```python
from build123d import *

# Parameters (mm, degrees)
SKETCH_1_W          = 35
SKETCH_1_H          = 35
SKETCH_1_R          = 1.7
EXTRUDE_1_DEPTH     = 8
SKETCH_2_W          = 5
SKETCH_2_H          = 8
EXTRUDE_2_DEPTH     = 40
SKETCH_3_R          = 1.6
CUT_EXTRUDE_1_DEPTH = 40
CUT_EXTRUDE_2_DEPTH = 24


with BuildPart() as part:
    # 草图1 → 凸台-拉伸1 (new body)
    with BuildSketch(Plane.XY):
        with Locations((6.7, -6.931428571)):
            Rectangle(SKETCH_1_W, SKETCH_1_H)
        with Locations((-4.8, 4.568571429)):
            Circle(SKETCH_1_R, mode=Mode.SUBTRACT)
        with Locations((18.2, 4.568571429)):
            Circle(SKETCH_1_R, mode=Mode.SUBTRACT)
        with Locations((-4.8, -18.431428571)):
            Circle(SKETCH_1_R, mode=Mode.SUBTRACT)
        with Locations((18.2, -18.431428571)):
            Circle(SKETCH_1_R, mode=Mode.SUBTRACT)
    extrude(amount=EXTRUDE_1_DEPTH)

    # 草图2 → 凸台-拉伸2 (add)
    with BuildSketch(Plane.XY.offset(8)):
        with Locations((-1.8, -6.931428571)):
            Rectangle(SKETCH_2_W, SKETCH_2_H)
        with Locations((15.2, -6.931428571)):
            Rectangle(SKETCH_2_W, SKETCH_2_H)
    extrude(amount=EXTRUDE_2_DEPTH)

    # 草图3 → 切除-拉伸1 (cut)
    with BuildSketch(Plane(origin=(17.7, 0, 0), x_dir=(0, 0, -1), z_dir=(1, 0, 0))):
        with Locations(Location((-38, -6.931428571, 0), (0, 0, 90))):
            Circle(SKETCH_3_R)
        with Locations(Location((-24, -6.931428571, 0), (0, 0, 90))):
            Circle(SKETCH_3_R)
    extrude(amount=-CUT_EXTRUDE_1_DEPTH, mode=Mode.SUBTRACT)

    # 草图5 → 切除-拉伸2 (cut)
    with BuildSketch(Plane.ZY.offset(4.3)):
        with BuildLine():
            Line((10.5, -6.931428571), (12, -6.931428571))
            Line((12, -6.931428571), (13.5, -6.931428571))
            ThreePointArc((13.5, -6.931428571), (12, -5.431428571), (10.5, -6.931428571))
        make_face()
        with BuildLine():
            Line((13.5, -6.931428571), (12, -6.931428571))
            Line((12, -6.931428571), (10.5, -6.931428571))
            ThreePointArc((10.5, -6.931428571), (12, -8.431428571), (13.5, -6.931428571))
        make_face()
        with BuildLine():
            ThreePointArc((45.5, -6.931428571), (44, -5.431428571), (42.5, -6.931428571))
            Line((42.5, -6.931428571), (44, -6.931428571))
            Line((44, -6.931428571), (45.5, -6.931428571))
        make_face()
        with BuildLine():
            Line((44, -6.931428571), (42.5, -6.931428571))
            ThreePointArc((42.5, -6.931428571), (44, -8.431428571), (45.5, -6.931428571))
            Line((45.5, -6.931428571), (44, -6.931428571))
        make_face()
    extrude(amount=-CUT_EXTRUDE_2_DEPTH, mode=Mode.SUBTRACT)


solid = part.part
```
Build history of the part. All positions in model axes, mm. A direction names the side the tool comes from. Round coordinates to 2 decimals unless told otherwise and drop trailing zeros. Order: outer loops, then holes, each group sorted by start corner. A loop starts at its lowest first (then second) coordinate and runs counter-clockwise, first axis right, second up. Notation, with made-up numbers: (73, 71.5) -> (88, 71.5) arc R21 cw to (88, 98.5) -> close; hole circle Ø3 at (15, -15). An arc over 180 degrees is marked (long way). Answer in a Markdown table with one row per item.
1) Wall check: L1, parallel to X at y = -4.5, z = 28.5; L2, parallel to Y at x = -4.8, z = 5; L3, parallel to Z at x = 5, y = -14.5. Give the ranges that are in metal, low to high.
Values:
| item | result |
|---|---|
| L1 | -4.3 to 0.7, 12.7 to 17.7 |
| L2 | -24.43 to -20.13, -16.73 to 2.87, 6.27 to 10.57 |
| L3 | 0 to 8 |
2) Band-saw the part on D-D on x = 13.5. Give the cut face in (y, z).
Values:
| item | result |
|---|---|
| outline | (-24.43, 0) -> (10.57, 0) -> (10.57, 8) -> (-2.93, 8) -> (-2.93, 48) -> (-10.93, 48) -> (-10.93, 8) -> (-24.43, 8) -> close; hole circle Ø3.2 at (-6.93, 24); hole circle Ø3.2 at (-6.93, 38); hole circle Ø3 at (-6.93, 12); hole circle Ø3 at (-6.93, 44) |
3) Band-saw the part on B-B on z = 35.5. Give the cut face in (x, y).
Values:
| item | result |
|---|---|
| outline | (-4.3, -10.93) -> (0.7, -10.93) -> (0.7, -2.93) -> (-4.3, -2.93) -> close; (12.7, -10.93) -> (17.7, -10.93) -> (17.7, -2.93) -> (12.7, -2.93) -> close |
4) Which spindle directions (+Z, -Z, +X, -X, +Y, -Y) get a long thin tool onto all of the face, cutting with end or side? Do faces 4 (the flat face through (0.7, -7, 28)), 5 (the flat face through (15, -2.931, 28)), 6 (the flat face through (-2, -10.931, 28)). Say none if no direction does.
Values:
| item | result |
|---|---|
| face 4 | +Z, +Y, -Y |
| face 5 | +Z, +X, -X, +Y |
| face 6 | +Z, +X, -X, -Y |
5) Band-saw the part on A-A on z = 24. Give the cut face in (x, y), and give its area (3 significant figures).
Values:
| item | result |
|---|---|
| outline | (-4.3, -10.93) -> (0.7, -10.93) -> (0.7, -8.53) -> (-4.3, -8.53) -> close; (-4.3, -5.33) -> (0.7, -5.33) -> (0.7, -2.93) -> (-4.3, -2.93) -> close; (12.7, -10.93) -> (17.7, -10.93) -> (17.7, -8.53) -> (12.7, -8.53) -> close; (12.7, -5.33) -> (17.7, -5.33) -> (17.7, -2.93) -> (12.7, -2.93) -> close |
| area | 48.0 mm2 |
6) Band-saw the part on C-C on y = 4. Give the cut face in (x, z), and give its area (3 significant figures).
Values:
| item | result |
|---|---|
| outline | (-10.8, 0) -> (-6.4, 0) -> (-6.4, 8) -> (-10.8, 8) -> close; (-3.2, 0) -> (16.6, 0) -> (16.6, 8) -> (-3.2, 8) -> close; (19.8, 0) -> (24.2, 0) -> (24.2, 8) -> (19.8, 8) -> close |
| area | 229 mm2 |
7) Pin check, flat tips, straight feed: P1, Ø9, axis at y = -8, z = 22.5, coming from the -X side; P2, Ø6, axis at x = 1.5, z = 22.5, coming from the -Y side; P3, Ø5.5, axis at x = -1.5, z = 22, coming from the +Y side. Stop position of each tip, or through.
Values:
| item | result |
|---|---|
| P1 | x = -4.3 |
| P2 | y = -10.93 |
| P3 | y = -2.93 |
8) Mould opens along X. For faces 1 (the flat face through (24.2, -7, 4)), 2 (the cylindrical face through (19.82, 5.08, 3.94)), 3 (the cylindrical face through (15.165, -7.945, 13.106)) say: released by +X, released by -X, zero draft, split by the parting line, or undercut.
Values:
| item | result |
|---|---|
| face 1 | released by +X |
| face 2 | undercut |
| face 3 | zero draft |
